Input: dimensioned drawing with shaded views. Units: mm. Origin: part minimum x, y, z. A direction names the side the tool comes from. Give positions to 0.01 mm unless a question says otherwise; leave off trailing zeros. Loops run counter-clockwise (first coordinate to the right, second up) from the corner with the lowest first, then second, coordinate; pieces in that order, holes last.
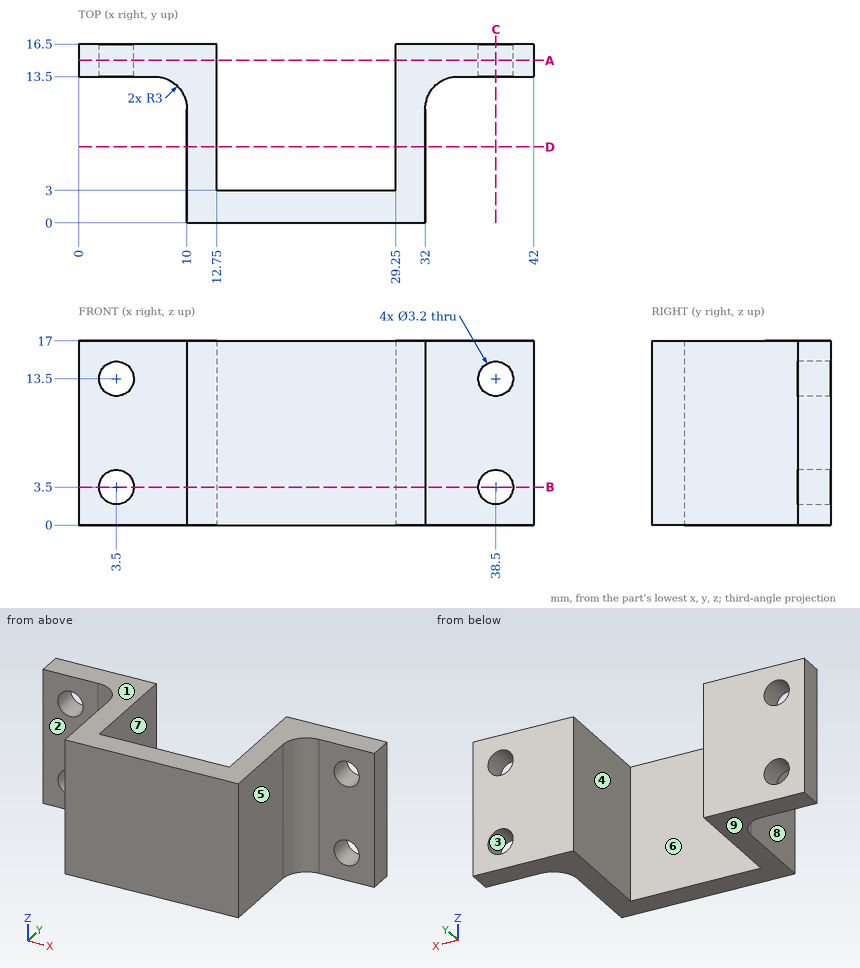
(1) Reachability of the marked faces 1, 2, 3, 4 and 5 from +Z, -Z, +X, -X, +Y, -Y: full face, straight path, thin tool, end or side. Return the list, or none.
A:
face 1: +Z, +X, -X, +Y, -Y
face 2: +Z, -Z, -X, -Y
face 3: +Y, -Y
face 4: +Z, -Z, +Y
face 5: +Z, -Z, +X, -Y
(2) Mould query, pull axis X, two halves, no side actions, for the marked faces 6, 7, 8 and 9. Classes: pulls with the +X half, pulls with the -X half, needs draft (parallel to the pull), parting line crosses it, or undercut.
A:
face 6: undercut
face 7: undercut
face 8: pulls with the -X half
face 9: needs draft
(3) Section C-C, the plane x = 38.5. Return the cut outline in (y, z).
A:
outline: (13.5, 0) - (16.5, 0) - (16.5, 1.9) - (13.5, 1.9) - close; (13.5, 5.1) - (16.5, 5.1) - (16.5, 11.9) - (13.5, 11.9) - close; (13.5, 15.1) - (16.5, 15.1) - (16.5, 17) - (13.5, 17) - close
(4) First-contact query: pin 1 (3.5 mm diameter, centred on x = 3, z = 6, fed in from -Y); pin 2 (4 mm diameter, centred on y = 7, z = 15, fed in from +X); pin 3 (1.5 mm diameter, centred on y = 2, z = 4, fed in from -X). Flat tips, straight axial feed; report the tip coordinate or a pass-through.
A:
pin 1: stops at y = 13.5
pin 2: stops at x = 32
pin 3: stops at x = 10
(5) Section A-A, the plane y = 15. Return the cut outline in (x, z).
A:
outline: (0, 0) - (12.75, 0) - (12.75, 17) - (0, 17) - close; (29.25, 0) - (42, 0) - (42, 17) - (29.25, 17) - close; hole circle Ø3.2 at (3.5, 3.5); hole circle Ø3.2 at (3.5, 13.5); hole circle Ø3.2 at (38.5, 3.5); hole circle Ø3.2 at (38.5, 13.5)
(6) Section D-D, the plane y = 7. Return the cut outline in (x, z), then the cut area to 3 significant figures.
A:
outline: (10, 0) - (12.75, 0) - (12.75, 17) - (10, 17) - close; (29.25, 0) - (32, 0) - (32, 17) - (29.25, 17) - close
area: 93.5 mm2
(7) Section B-B, the plane z = 3.5. Return the cut outline in (x, y).
A:
outline: (0, 13.5) - (1.9, 13.5) - (1.9, 16.5) - (0, 16.5) - close; (5.1, 13.5) - (7, 13.5) arc R3 cw to (10, 10.5) - (10, 0) - (32, 0) - (32, 10.5) arc R3 cw to (35, 13.5) - (36.9, 13.5) - (36.9, 16.5) - (29.25, 16.5) - (29.25, 3) - (12.75, 3) - (12.75, 16.5) - (5.1, 16.5) - close; (40.1, 13.5) - (42, 13.5) - (42, 16.5) - (40.1, 16.5) - close
(8) Ray query, line 1 along X through (y, z) = (15.05, 13.5); line 2 along X through (y, z) = (4.5, 14); line 3 along Y through (x, z) = (24.5, 14). Return the intervals inside material, ascending.
A:
line 1: x = 0 to 1.9, 5.1 to 12.75, 29.25 to 36.9, 40.1 to 42
line 2: x = 10 to 12.75, 29.25 to 32
line 3: y = 0 to 3
